```python
from build123d import *

# Parameters (mm, degrees)
F0_R            = 25
F0_R_2          = 2.25
F1_DEPTH        = 14
F2_DEPTH        = 10
F4_DEPTH        = 14.001
F5_R            = 3
F7_DEPTH        = 12
F7_COPIES_COUNT = 4


# Not quite as in the source:
# - a pattern or mirror of a feature is missing from the dataset's text; its kind, count and spacing are read off the source's solid


with BuildPart() as f1:
    # F0 (on Top) → F1 (new body)
    with BuildSketch(Plane.XY):
        with BuildLine():
            ThreePointArc((57, 18.7349939952), (42.4264068712, 42.4264068712), (18.7349939952, 57))
            Line((18.7349939952, 57), (-18.7349939952, 57))
            ThreePointArc((-18.7349939952, 57), (-42.4264068712, 42.4264068712), (-57, 18.7349939952))
            Line((-57, 18.7349939952), (-57, -18.7349939952))
            ThreePointArc((-57, -18.7349939952), (-42.4264068712, -42.4264068712), (-18.7349939952, -57))
            Line((-18.7349939952, -57), (18.7349939952, -57))
            ThreePointArc((18.7349939952, -57), (42.4264068712, -42.4264068712), (57, -18.7349939952))
            Line((57, -18.7349939952), (57, 18.7349939952))
        make_face()
        Circle(F0_R, mode=Mode.SUBTRACT)
        Circle(F0_R)
        with BuildLine():
            ThreePointArc((-18.7349939952, 57), (-9.486832838, 59.2452529972), (2.885e-07, 60))
            Line((2.885e-07, 60), (-52, 60))
            ThreePointArc((-52, 60), (-57.6568542495, 57.6568542495), (-60, 52))
            Line((-60, 52), (-60, 2.895e-07))
            ThreePointArc((-60, 2.895e-07), (-59.2452529515, 9.4868331234), (-57, 18.7349939952))
            ThreePointArc((-57, 18.7349939952), (-42.4264068712, 42.4264068712), (-18.7349939952, 57))
        make_face()
        with Locations((-52.5, 52.5)):
            Circle(F0_R_2, mode=Mode.SUBTRACT)
        with BuildLine():
            ThreePointArc((-57, -18.7349939952), (-59.2452529973, -9.4868328376), (-60, 2.895e-07))
            Line((-60, 2.895e-07), (-60, -52))
            ThreePointArc((-60, -52), (-57.6568542495, -57.6568542495), (-52, -60))
            Line((-52, -60), (-2.57e-07, -60))
            ThreePointArc((-2.57e-07, -60), (-9.4868331074, -59.2452529541), (-18.7349939952, -57))
            ThreePointArc((-18.7349939952, -57), (-42.4264068712, -42.4264068712), (-57, -18.7349939952))
        make_face()
        with Locations((-52.5, -52.5)):
            Circle(F0_R_2, mode=Mode.SUBTRACT)
        with BuildLine():
            Line((60, -52), (60, 0))
            ThreePointArc((60, 0), (59.2452529744, -9.4868329805), (57, -18.7349939952))
            ThreePointArc((57, -18.7349939952), (42.4264068712, -42.4264068712), (18.7349939952, -57))
            ThreePointArc((18.7349939952, -57), (9.4868328536, -59.2452529947), (-2.57e-07, -60))
            Line((-2.57e-07, -60), (52, -60))
            ThreePointArc((52, -60), (57.6568542495, -57.6568542495), (60, -52))
        make_face()
        with Locations((52.5, -52.5)):
            Circle(F0_R_2, mode=Mode.SUBTRACT)
        with BuildLine():
            ThreePointArc((60, 52), (57.6568542495, 57.6568542495), (52, 60))
            Line((52, 60), (2.885e-07, 60))
            ThreePointArc((2.885e-07, 60), (9.486833123, 59.2452529516), (18.7349939952, 57))
            ThreePointArc((18.7349939952, 57), (42.4264068712, 42.4264068712), (57, 18.7349939952))
            ThreePointArc((57, 18.7349939952), (59.2452529744, 9.4868329805), (60, 0))
            Line((60, 0), (60, 52))
        make_face()
        with Locations((52.5, 52.5)):
            Circle(F0_R_2, mode=Mode.SUBTRACT)
        with BuildLine():
            ThreePointArc((18.7349939952, 57), (9.486833123, 59.2452529516), (2.885e-07, 60))
            ThreePointArc((2.885e-07, 60), (-9.486832838, 59.2452529972), (-18.7349939952, 57))
            Line((-18.7349939952, 57), (18.7349939952, 57))
        make_face()
        with BuildLine():
            Line((-57, -18.7349939952), (-57, 18.7349939952))
            ThreePointArc((-57, 18.7349939952), (-59.2452529515, 9.4868331234), (-60, 2.895e-07))
            ThreePointArc((-60, 2.895e-07), (-59.2452529973, -9.4868328376), (-57, -18.7349939952))
        make_face()
        with BuildLine():
            ThreePointArc((-2.57e-07, -60), (9.4868328536, -59.2452529947), (18.7349939952, -57))
            Line((18.7349939952, -57), (-18.7349939952, -57))
            ThreePointArc((-18.7349939952, -57), (-9.4868331074, -59.2452529541), (-2.57e-07, -60))
        make_face()
        with BuildLine():
            ThreePointArc((57, -18.7349939952), (59.2452529744, -9.4868329805), (60, 0))
            ThreePointArc((60, 0), (59.2452529744, 9.4868329805), (57, 18.7349939952))
            Line((57, 18.7349939952), (57, -18.7349939952))
        make_face()
    extrude(amount=F1_DEPTH)

    # F0 (on Top) → F2 (cut)
    with BuildSketch(Plane.XY):
        with BuildLine():
            ThreePointArc((57, 18.7349939952), (42.4264068712, 42.4264068712), (18.7349939952, 57))
            Line((18.7349939952, 57), (-18.7349939952, 57))
            ThreePointArc((-18.7349939952, 57), (-42.4264068712, 42.4264068712), (-57, 18.7349939952))
            Line((-57, 18.7349939952), (-57, -18.7349939952))
            ThreePointArc((-57, -18.7349939952), (-42.4264068712, -42.4264068712), (-18.7349939952, -57))
            Line((-18.7349939952, -57), (18.7349939952, -57))
            ThreePointArc((18.7349939952, -57), (42.4264068712, -42.4264068712), (57, -18.7349939952))
            Line((57, -18.7349939952), (57, 18.7349939952))
        make_face()
        Circle(F0_R, mode=Mode.SUBTRACT)
        Circle(F0_R)
    extrude(amount=F2_DEPTH, mode=Mode.SUBTRACT)

    # F3 (on face) → F4 (cut, through all)
    with BuildSketch(Plane.XY):
        with BuildLine():
            ThreePointArc((51.9615242271, -30), (54.7711468799, -24.4973767873), (57, -18.7349939952))
            Line((57, -18.7349939952), (57, 1.314733996))
            ThreePointArc((57, 1.314733996), (22.5078780664, -33.1091892137), (-21.6506350946, -12.5))
            ThreePointArc((-21.6506350946, -12.5), (-25, 0), (-21.6506350946, 12.5))
            ThreePointArc((-21.6506350946, 12.5), (-6.0945554338, -45.5560796608), (51.9615242271, -30))
        make_face()
        with BuildLine():
            Line((-18.7349939952, -57), (1.314733996, -57))
            ThreePointArc((1.314733996, -57), (-33.1091892137, -22.5078780664), (-12.5, 21.6506350946))
            ThreePointArc((-12.5, 21.6506350946), (0, 25), (12.5, 21.6506350946))
            ThreePointArc((12.5, 21.6506350946), (-45.5560796608, 6.0945554338), (-30, -51.9615242271))
            ThreePointArc((-30, -51.9615242271), (-24.4973767873, -54.7711468799), (-18.7349939952, -57))
        make_face()
        with BuildLine():
            ThreePointArc((-12.5, -21.6506350946), (45.5560796608, -6.0945554338), (30, 51.9615242271))
            ThreePointArc((30, 51.9615242271), (24.4973767873, 54.7711468799), (18.7349939952, 57))
            Line((18.7349939952, 57), (-1.314733996, 57))
            ThreePointArc((-1.314733996, 57), (33.1091892137, 22.5078780664), (12.5, -21.6506350946))
            ThreePointArc((12.5, -21.6506350946), (0, -25), (-12.5, -21.6506350946))
        make_face()
        with BuildLine():
            ThreePointArc((25, 0), (24.1481456572, -6.4704761276), (21.6506350946, -12.5))
            ThreePointArc((21.6506350946, -12.5), (6.0945554338, 45.5560796608), (-51.9615242271, 30))
            ThreePointArc((-51.9615242271, 30), (-54.7711468799, 24.4973767873), (-57, 18.7349939952))
            Line((-57, 18.7349939952), (-57, -1.314733996))
            ThreePointArc((-57, -1.314733996), (-22.5078780664, 33.1091892137), (21.6506350946, 12.5))
            ThreePointArc((21.6506350946, 12.5), (24.1481456572, 6.4704761276), (25, 0))
        make_face()
    extrude(amount=F4_DEPTH, mode=Mode.SUBTRACT)

    # F5
    f5_edges = [f1.edges().sort_by_distance(p)[0] for p in [
        (21.650635, -12.5, 12),
        (12.5, 21.650635, 12),
        (-21.650635, 12.5, 12),
        (-12.5, -21.650635, 12),
        (-57, -1.314734, 12),
        (-1.314734, 57, 12),
        (57, 1.314734, 12),
        (1.314734, -57, 12),
    ]]
    fillet(f5_edges, radius=F5_R)

    # F6 (on face) → F7 (cut)
    with BuildSketch(Plane.XY):
        with BuildLine():
            ThreePointArc((58, -21.9089023002), (43.8406204336, -43.8406204336), (21.9089023002, -58))
            Line((21.9089023002, -58), (48.1010791024, -58))
            ThreePointArc((48.1010791024, -58), (49.0271170017, -57.3774305355), (48.8001090628, -56.2849076182))
            ThreePointArc((48.8001090628, -56.2849076182), (48.7573593129, -48.7573593129), (56.2849076182, -48.8001090628))
            ThreePointArc((56.2849076182, -48.8001090628), (57.3774305355, -49.0271170017), (58, -48.1010791024))
            Line((58, -48.1010791024), (58, -21.9089023002))
        make_face()
    f7 = extrude(amount=F7_DEPTH, mode=Mode.SUBTRACT)

    # F7_copies: F7 ×4 about axis
    f7_copies_axis = Axis((0, 0, 0), (0, 0, 1))
    for i in range(1, F7_COPIES_COUNT):
        add(f7.rotate(f7_copies_axis, i * 360 / F7_COPIES_COUNT), mode=Mode.SUBTRACT)


solid = f1.part
```
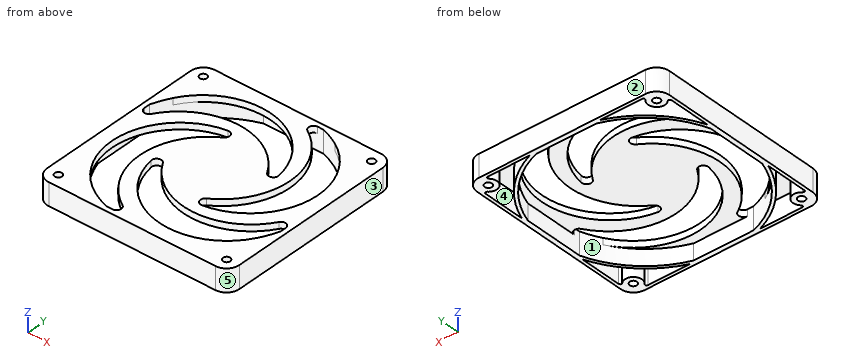
Read the model definition and answer for the solid it produces. Units are mm, in the model's axes. Face numbers are marked on the shaded views. A direction names the side the tool comes from. Give positions to 0.01 mm unless a question says otherwise; leave off trailing zeros. Write each loop counter-clockwise with the first axis right and the second up, starting at its lowest first coordinate (ties: lowest second). Pieces come first, ordered by that corner, then holes. Notation, with made-up numbers: M 5.25,48 L 54.25,48 A33 ccw 54.25,82 Z; hole C 55.25,47 d4. An arc over 180 degrees is marked long. Put each result on its own line as item: value. Start each with the question number.
1. Consider line 1 along X through (y, z) = (-7, 5.5); line 2 along Y through (x, z) = (-52.5, 3.5). Determine where each line is inside the solid, lowest interval first.
2. The part is cut by section C-C, the plane x = 40. Give the vertices of the cut face in (y, z), and give its area (3 significant figures).
3. Which of the six approach directions +Z, -Z, +X, -X, +Y, -Y give full straight-line access (tool end or side, diameter ignored) to the marked faces 4 and 5?
4. The part is cut by section D-D, the plane z = 7.5. Give the number of separate pieces and of enclosed holes in the cut face, and give its area (3 significant figures).
5. The part is cut by section A-A, the plane y = -42. Give the vertices of the cut face in (x, z), and give its area (3 significant figures).
6. The part is cut by section B-B, the plane y = -28.5. Give the vertices of the cut face in (x, z), and give its area (3 significant figures).
7. For a pull along X with two mould halves and no side action, classify the marked faces 1, 2 and 3 as released by +X, released by -X, zero draft, split by the parting line, or undercut.
8. Each of these flat-tipped pins is pushed along its axis until it touches: pin 1 Ø5 at (x, y) = (-41.5, 22) entering from -Z; pin 2 Ø2.5 at (x, y) = (52.5, -52.5) entering from -Z; pin 3 Ø6 at (x, y) = (-52.5, 52.5) entering from +Z. Where does it stop, or does it pass through?
Final values:
1. line 1: x = -60 to -57, 57 to 60
1. line 2: y = -59.98 to -54.75, -50.25 to -47.21, -32.98 to -29.05, 29.05 to 32.98, 47.21 to 50.25, 54.75 to 59.98
2. outline: M -60,0 L -58,0 L -58,12 L -47.37,12 L -47.37,0 L -44.72,0 L -44.72,10 L -43.23,10 L -43.23,14 L -60,14 Z; M -25.73,10 L -13.65,10 L -13.65,14 L -25.73,14 Z; M 43.96,10 L 44.72,10 L 44.72,0 L 47.37,0 L 47.37,12 L 58,12 L 58,0 L 60,0 L 60,14 L 43.96,14 Z
2. area: 230 mm²
3. face 4: -Z
3. face 5: +Z, -Z, +X, -Y
4. separate pieces: 1
4. enclosed holes: 9
4. area: 1,830 mm²
5. outline: M -60,0 L -58,0 L -58,12 L -45.61,12 L -45.61,0 L -42.85,0 L -42.85,10 L -41.7,10 L -41.7,14 L -60,14 Z; M -24.2,10 L -11.32,10 L -11.32,14 L -24.2,14 Z; M 41.63,10 L 42.85,10 L 42.85,0 L 45.61,0 L 45.61,12 L 58,12 L 58,0 L 60,0 L 60,14 L 41.63,14 Z
5. area: 244 mm²
6. outline: M -60,0 L -58,0 L -58,12 L -55.06,12 L -55.06,0 L -52.8,0 L -52.8,10 L -49.1,10 L -49.1,14 L -60,14 Z; M -31.6,10 L -22.48,10 L -22.48,14 L -31.6,14 Z; M -5.31,10 L 35.62,10 L 35.62,14 L -5.31,14 Z; M 52.8,0 L 55.06,0 L 55.06,12 L 58,12 L 58,0 L 60,0 L 60,14 L 52.8,14 Z
6. area: 346 mm²
7. face 1: undercut
7. face 2: zero draft
7. face 3: released by +X
8. pin 1: stops at z = 10
8. pin 2: passes through
8. pin 3: stops at z = 14
